Here's how the part is built. I have some questions about the finished solid (model axes, mm). Face numbers are marked on the shaded views. A direction names the side the tool comes from. Round coordinates to 2 decimals unless told otherwise and drop trailing zeros. Write each loop counter-clockwise with the first axis right and the second up, starting at its lowest first coordinate (ties: lowest second). Pieces come first, ordered by that corner, then holes. Notation, with made-up numbers: M 9.5,64 L 40.5,64 A29 cw 40.5,95 Z; hole C 4.25,82.25 d11. An arc over 180 degrees is marked long. Write item = value, one per line. Start each with the question number.
(1) I want a section at A-A (z = 0). List the corners of the cut face in (x, y) for me (3 decimals).
(2) If we mould it in two halves opening along Z, with no side actions, what happens to the marked faces 3, 4, 5 and 6? For each: released by +Z, released by -Z, zero draft, split by the parting line, or undercut.
(3) On a 3-axis mill with a long thin cutter (end or side, diameter ignored), from which of +Z, -Z, +X, -X, +Y, -Y can I reach the whole of each face in a straight line? I mean the marked faces 1 and 2. Say none if no direction works.
(4) I want a section at C-C (x = 14.5). List the corners of the cut face in (y, z) for me (3 decimals), and give its area (3 significant figures).
(5) Will these pins go through, and if not, where does the flat tip stop? pin 1 Ø1.4 at (y, z) = (4, 9) entering from -X; pin 2 Ø10 at (x, z) = (4.5, 1) entering from +Y; pin 3 Ø4 at (x, z) = (26.64, -6.5) entering from -Y; pin 4 Ø0.6 at (y, z) = (4, -8.5) entering from +X.
(6) I want a section at D-D (x = 7). List the corners of the cut face in (y, z) for me (3 decimals), and give its area (3 significant figures).
(7) I need wall thicknesses on line 1 along X through (y, z) = (-0.6, 0) (3 decimals); line 2 along Z through (x, y) = (18, 12) (3 decimals); line 3 along Y through (x, z) = (28.5, -7.5). Which ranges of each line are inside material? Lowest first, please.
(8) I want a section at B-B (y = 5.75). List the corners of the cut face in (x, z) for me (3 decimals), and give its area (3 significant figures).
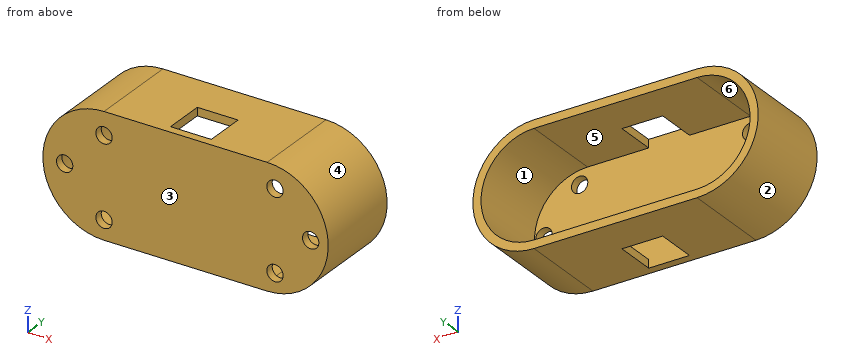
```python
from build123d import *

# Parameters (mm, degrees)
BOSS_EXTRUDE1_DEPTH = 12.7
BOSS_EXTRUDE2_START = 1.27
BOSS_EXTRUDE2_DEPTH = 1.27
SKETCH4_W           = 6.35
SKETCH4_H           = 6.35
CUT_EXTRUDE1_DEPTH  = 42.760604941
CUT_EXTRUDE2_REACH  = 40.364
SKETCH5_R           = 1.27


with BuildPart() as part:
    # Sketch2 → Boss-Extrude1 (new body)
    with BuildSketch(Plane(origin=(0, 0, 0), x_dir=(1, 0, 0), z_dir=(0, 1, 0))):
        with BuildLine():
            Line((0, 9.525), (25.4, 9.525))
            ThreePointArc((25.4, 9.525), (34.925, 0), (25.4, -9.525))
            Line((25.4, -9.525), (0, -9.525))
            ThreePointArc((0, -9.525), (-9.525, 0), (0, 9.525))
        make_face()
        with BuildLine():
            Line((0, 8.255), (25.4, 8.255))
            ThreePointArc((25.4, 8.255), (33.655, 0), (25.4, -8.255))
            Line((25.4, -8.255), (0, -8.255))
            ThreePointArc((0, -8.255), (-8.255, 0), (0, 8.255))
        make_face(mode=Mode.SUBTRACT)
    extrude(amount=BOSS_EXTRUDE1_DEPTH)

    # Sketch3 → Boss-Extrude2 (add)
    with BuildSketch(Plane.XZ.offset(BOSS_EXTRUDE2_START)):
        with BuildLine():
            Line((0, 9.525), (25.4, 9.525))
            ThreePointArc((25.4, 9.525), (34.925, 0), (25.4, -9.525))
            Line((25.4, -9.525), (0, -9.525))
            ThreePointArc((0, -9.525), (-9.525, 0), (0, 9.525))
        make_face()
    extrude(amount=-BOSS_EXTRUDE2_DEPTH)

    # Sketch4 → Cut-Extrude1 (cut, through all)
    with BuildSketch(Plane.XY.offset(9.525)):
        with Locations((12.7, 3.175)):
            Rectangle(SKETCH4_W, SKETCH4_H)
    extrude(amount=-CUT_EXTRUDE1_DEPTH, mode=Mode.SUBTRACT)

    # Sketch5 → Cut-Extrude2 (cut, up to next)
    with BuildSketch(Plane(origin=(0, 0, 0), x_dir=(1, 0, 0), z_dir=(0, 1, 0)), mode=Mode.PRIVATE) as cut_extrude2_sk1:
        with Locations(Location((-6.12696281, 0, 0), (0, 0, 270))):
            Circle(SKETCH5_R)
    cut_extrude2_tool1 = extrude(cut_extrude2_sk1.sketch, amount=-CUT_EXTRUDE2_REACH, mode=Mode.PRIVATE) & part.part
    # Sketch5 → Cut-Extrude2 (cut, up to next)
    with BuildSketch(Plane(origin=(0, 0, 0), x_dir=(1, 0, 0), z_dir=(0, 1, 0)), mode=Mode.PRIVATE) as cut_extrude2_sk2:
        with Locations(Location((32.190803921, 0, 0), (0, 0, 270))):
            Circle(SKETCH5_R)
    cut_extrude2_tool2 = extrude(cut_extrude2_sk2.sketch, amount=-CUT_EXTRUDE2_REACH, mode=Mode.PRIVATE) & part.part
    # Sketch5 → Cut-Extrude2 (cut, up to next)
    with BuildSketch(Plane(origin=(0, 0, 0), x_dir=(1, 0, 0), z_dir=(0, 1, 0)), mode=Mode.PRIVATE) as cut_extrude2_sk3:
        with Locations(Location((0, 6.499696211, 0), (0, 0, 270))):
            Circle(SKETCH5_R)
    cut_extrude2_tool3 = extrude(cut_extrude2_sk3.sketch, amount=-CUT_EXTRUDE2_REACH, mode=Mode.PRIVATE) & part.part
    # Sketch5 → Cut-Extrude2 (cut, up to next)
    with BuildSketch(Plane(origin=(0, 0, 0), x_dir=(1, 0, 0), z_dir=(0, 1, 0)), mode=Mode.PRIVATE) as cut_extrude2_sk4:
        with Locations(Location((0, -5.991753651, 0), (0, 0, 270))):
            Circle(SKETCH5_R)
    cut_extrude2_tool4 = extrude(cut_extrude2_sk4.sketch, amount=-CUT_EXTRUDE2_REACH, mode=Mode.PRIVATE) & part.part
    # Sketch5 → Cut-Extrude2 (cut, up to next)
    with BuildSketch(Plane(origin=(0, 0, 0), x_dir=(1, 0, 0), z_dir=(0, 1, 0)), mode=Mode.PRIVATE) as cut_extrude2_sk5:
        with Locations(Location((26.63537738, 6.499696211, 0), (0, 0, 270))):
            Circle(SKETCH5_R)
    cut_extrude2_tool5 = extrude(cut_extrude2_sk5.sketch, amount=-CUT_EXTRUDE2_REACH, mode=Mode.PRIVATE) & part.part
    # Sketch5 → Cut-Extrude2 (cut, up to next)
    with BuildSketch(Plane(origin=(0, 0, 0), x_dir=(1, 0, 0), z_dir=(0, 1, 0)), mode=Mode.PRIVATE) as cut_extrude2_sk6:
        with Locations(Location((26.63537738, -5.991753651, 0), (0, 0, 270))):
            Circle(SKETCH5_R)
    cut_extrude2_tool6 = extrude(cut_extrude2_sk6.sketch, amount=-CUT_EXTRUDE2_REACH, mode=Mode.PRIVATE) & part.part
    add(cut_extrude2_tool1.solids().sort_by_distance((-6.126963, 0, 0))[0], mode=Mode.SUBTRACT)
    add(cut_extrude2_tool2.solids().sort_by_distance((32.190804, 0, 0))[0], mode=Mode.SUBTRACT)
    add(cut_extrude2_tool3.solids().sort_by_distance((0, 0, -6.499696))[0], mode=Mode.SUBTRACT)
    add(cut_extrude2_tool4.solids().sort_by_distance((0, 0, 5.991754))[0], mode=Mode.SUBTRACT)
    add(cut_extrude2_tool5.solids().sort_by_distance((26.635377, 0, -6.499696))[0], mode=Mode.SUBTRACT)
    add(cut_extrude2_tool6.solids().sort_by_distance((26.635377, 0, 5.991754))[0], mode=Mode.SUBTRACT)


solid = part.part
```
Returned:
q1.outline = M -9.525,-1.27 L -7.397,-1.27 L -7.397,0 L -8.255,0 L -8.255,12.7 L -9.525,12.7 Z; M -4.857,-1.27 L 30.921,-1.27 L 30.921,0 L -4.857,0 Z; M 33.461,-1.27 L 34.925,-1.27 L 34.925,12.7 L 33.655,12.7 L 33.655,0 L 33.461,0 Z
q2.face_3 = zero draft
q2.face_4 = split by the parting line
q2.face_5 = undercut
q2.face_6 = undercut
q3.face_1 = +Y
q3.face_2 = -X, +Y, -Y
q4.outline = M -1.27,-9.525 L 0,-9.525 L 0,9.525 L -1.27,9.525 Z; M 6.35,-9.525 L 12.7,-9.525 L 12.7,-8.255 L 6.35,-8.255 Z; M 6.35,8.255 L 12.7,8.255 L 12.7,9.525 L 6.35,9.525 Z
q4.area = 40.3 mm²
q5.pin_1 = -4.67
q5.pin_2 = 0
q5.pin_3 = -1.27
q5.pin_4 = 30.25
q6.outline = M -1.27,-9.525 L 12.7,-9.525 L 12.7,-8.255 L 0,-8.255 L 0,8.255 L 12.7,8.255 L 12.7,9.525 L -1.27,9.525 Z
q6.area = 56.5 mm²
q7.line_1 = -9.525 to -7.397, -4.857 to 30.921, 33.461 to 34.925
q7.line_2 = -9.525 to -8.255, 8.255 to 9.525
q7.line_3 = -1.27 to 0
q8.outline = M 0,-9.525 L 9.525,-9.525 L 9.525,-8.255 L 0,-8.255 A8.255 cw 0,8.255 L 9.525,8.255 L 9.525,9.525 L 0,9.525 A9.525 ccw Z; M 15.875,-9.525 L 25.4,-9.525 A9.525 ccw 25.4,9.525 L 15.875,9.525 L 15.875,8.255 L 25.4,8.255 A8.255 cw 25.4,-8.255 L 15.875,-8.255 Z
q8.area = 119 mm²
